```python
from build123d import *

# Parameters (mm, degrees)
F0_W     = 254
F0_H     = 152.4
F1_DEPTH = 101.6
F2_W     = 152.4
F2_H     = 77.6838691145
F3_DEPTH = 215.9
F4_W     = 25.4
F4_H     = 25.4
F5_DEPTH = 50.8
F8_DEPTH = 25.4
F6_R     = 37.2654170077
F9_DEPTH = 25.4


with BuildPart() as f1:
    # F0 (on Top) → F1 (new body)
    with BuildSketch(Plane.XY):
        with Locations((111.9955861747, 48.1005767256)):
            Rectangle(F0_W, F0_H)
    extrude(amount=F1_DEPTH)

    # F2 (on face) → F3 (cut)
    with BuildSketch(Plane(origin=(-15.0044138253, 0, 0), x_dir=(0, -1, 0), z_dir=(-1, 0, 0))):
        with Locations((-48.1005767256, 62.7580654427)):
            Rectangle(F2_W, F2_H)
    extrude(amount=-F3_DEPTH, mode=Mode.SUBTRACT)

    # F4 (on face) → F5 (cut)
    with BuildSketch(Plane(origin=(200.8955861747, 0, 0), x_dir=(0, -1, 0), z_dir=(-1, 0, 0))):
        with Locations((-111.6005767256, 88.9)):
            Rectangle(F4_W, F4_H)
    extrude(amount=-F5_DEPTH, mode=Mode.SUBTRACT)

    # F7 (on face) → F8 (cut)
    with BuildSketch(Plane.XY.offset(23.9161308855)):
        with BuildLine():
            ThreePointArc((43.4155861747, -28.0994232744), (-13.8048519796, 48.1005767256), (43.4155861747, 124.3005767256))
            Line((43.4155861747, 124.3005767256), (-15.0044138253, 124.3005767256))
            Line((-15.0044138253, 124.3005767256), (-15.0044138253, -28.0994232744))
            Line((-15.0044138253, -28.0994232744), (43.4155861747, -28.0994232744))
        make_face()
    extrude(amount=-F8_DEPTH, mode=Mode.SUBTRACT)

    # F6 (on face) → F9 (cut)
    with BuildSketch(Plane.XY.offset(23.9161308855)):
        with Locations((73.0605365211, 48.3872703384)):
            Circle(F6_R)
    extrude(amount=-F9_DEPTH, mode=Mode.SUBTRACT)


solid = f1.part
```
The listing builds one solid part. Answer for the finished solid, in the listing's coordinates (mm). A direction names the side the tool comes from. Give positions to 0.01 mm unless a question says otherwise; leave off trailing zeros. Order: outer loops, then holes, each group sorted by start corner. A loop starts at its lowest first (then second) coordinate and runs counter-clockwise, first axis right, second up. Notation, with made-up numbers: (57.5, -39.75) -> (77.5, -39.75) arc R22 ccw to (77.5, -4.75) -> close; hole circle Ø6 at (-26.5, 77). An arc over 180 degrees is marked (long way). Answer as CSV lines item,"result". Start each with the question number.
Q1. A cutting plane is placed at A-A (y = 57.5). Determine the outline of the cut face in (x, z).
Q2. A cutting plane is placed at C-C (x = 96). Determine the outline of the cut face in (y, z).
Q3. A cutting plane is placed at D-D (x = 222). Determine the outline of the cut face in (y, z).
Q4. Given pin 1 (1 mm diameter, centred on y = 20.5, z = 51, fed in from -X); pin 2 (7.5 mm diameter, centred on x = 217.5, y = 109, fed in from +Z); pin 3 (4 mm diameter, centred on x = 199.5, y = 26.5, fed in from -Z); pin 4 (1 mm diameter, centred on y = 60, z = 16.5, fed in from -X), each flat-ended and moving along its own axis, determine where each tip first touches the part or whether it passes through.
Q5. Determine the mould class of faces 3 (the cylindrical face through (43.49, 25.71, 12.13)), 4 (the flat face through (220, 98.901, 89)), 5 (the flat face through (183, -28.099, 16)), 6 (the flat face through (220, 112, 76.2)) for opening direction Y: pulls with the +Y half, pulls with the -Y half, needs draft (parallel to the pull), parting line crosses it, or undercut.
Q6. A cutting plane is placed at B-B (z = 13). Determine the outline of the cut face in (x, y), then the cut area to 3 significant figures.
Q7. Which of the six approach directions +Z, -Z, +X, -X, +Y, -Y give full straight-line access (tool end or side, diameter ignored) to faces 1 (the flat face through (162, 124.301, 21)), 2 (the flat face through (116, 49, 23.916))?
Q8. Find the intervals of material crossed by L1, parallel to X at y = 41.5, z = 66; L2, parallel to Z at x = 138, y = 5; L3, parallel to X at y = 108, z = 13, in increasing order.
Results found:
1,outline,"(-13.25, 0) -> (36.93, 0) -> (36.93, 23.92) -> (-13.25, 23.92) -> close; (109.19, 0) -> (239, 0) -> (239, 101.6) -> (200.9, 101.6) -> (200.9, 23.92) -> (109.19, 23.92) -> close"
2,outline,"(-28.1, 0) -> (19.02, 0) -> (19.02, 23.92) -> (-28.1, 23.92) -> close; (77.76, 0) -> (124.3, 0) -> (124.3, 23.92) -> (77.76, 23.92) -> close"
3,outline,"(-28.1, 0) -> (124.3, 0) -> (124.3, 76.2) -> (98.9, 76.2) -> (98.9, 101.6) -> (-28.1, 101.6) -> close"
4,pin 1,"x = 200.9"
4,pin 2,"z = 76.2"
4,pin 3,"z = 0"
4,pin 4,"x = -12.98"
5,face 3,"undercut"
5,face 4,"pulls with the +Y half"
5,face 5,"pulls with the -Y half"
5,face 6,"needs draft"
6,outline,"(43.42, -28.1) -> (239, -28.1) -> (239, 124.3) -> (43.42, 124.3) arc R79.35 ccw to start; hole circle Ø74.53 at (73.06, 48.39)"
6,area,"31,900 mm2"
7,face 1,"+Z, -Z, +X, -X, +Y"
7,face 2,"+Z, -X, +Y, -Y"
8,L1,"200.9 to 239"
8,L2,"0 to 23.92"
8,L3,"13.5 to 239"
